```python
from build123d import *

# Parameters (mm, degrees)
F0_W     = 22
F0_H     = 55
F1_DEPTH = 3
F2_R     = 2
F4_DEPTH = 2
F5_R     = 4
F6_R     = 19
F6_R_2   = 16.5
F7_DEPTH = 15
F9_DEPTH = 25


with BuildPart() as f1:
    # F0 (on Top) → F1 (new body)
    with BuildSketch(Plane.XY):
        Rectangle(F0_W, F0_H)
    extrude(amount=F1_DEPTH)

    # F2
    f2_edges = [f1.edges().sort_by_distance(p)[0] for p in [
        (-11, 27.5, 1.5),
        (11, 27.5, 1.5),
        (11, -27.5, 1.5),
        (-11, -27.5, 1.5),
    ]]
    fillet(f2_edges, radius=F2_R)

    # F3 (on face) → F4 (join)
    with BuildSketch(Plane.XZ.offset(27.5)):
        with BuildLine():
            Line((-9, 3), (-4.24e-08, 3))
            Line((-4.24e-08, 3), (9, 3))
            Line((9, 3), (9, 2.7667994693))
            ThreePointArc((9, 2.7667994693), (16.3095064303, 9.7532056552), (19, 19.5))
            ThreePointArc((19, 19.5), (-9.7467943448, 35.8095064303), (-9, 2.7667994693))
            Line((-9, 2.7667994693), (-9, 3))
        make_face()
        with BuildLine():
            ThreePointArc((-4.24e-08, 3), (-11.6672618746, 31.1672619046), (16.5, 19.5))
            ThreePointArc((16.5, 19.5), (11.6672618746, 7.8327380954), (-4.24e-08, 3))
        make_face(mode=Mode.SUBTRACT)
        with BuildLine():
            ThreePointArc((-4.24e-08, 3), (11.6672618746, 7.8327380954), (16.5, 19.5))
            ThreePointArc((16.5, 19.5), (-11.6672618746, 31.1672619046), (-4.24e-08, 3))
        make_face()
    extrude(amount=-F4_DEPTH)

    # F5
    f5_edges = [f1.edges().sort_by_distance(p)[0] for p in [
        (0, -25.5, 3),
    ]]
    fillet(f5_edges, radius=F5_R)

    # F6 (on face) → F7 (join)
    with BuildSketch(Plane(origin=(0, 27.5, 0), x_dir=(-1, 0, 0), z_dir=(0, 1, 0))):
        with Locations((0, 19.5)):
            Circle(F6_R)
        with Locations((0, 19.5)):
            Circle(F6_R_2, mode=Mode.SUBTRACT)
    extrude(amount=-F7_DEPTH)

    # F8 (on face) → F9 (cut)
    with BuildSketch(Plane(origin=(0, 27.5, 0), x_dir=(-1, 0, 0), z_dir=(0, 1, 0))):
        Polygon((-10.5, 26.4886836855), (0, 26.4886836855), (10.5, 26.4886836855), (23.2279220614, 39.2166057468), (-23.2279220614, 39.2166057468), align=None)
    extrude(amount=-F9_DEPTH, mode=Mode.SUBTRACT)


solid = f1.part
```
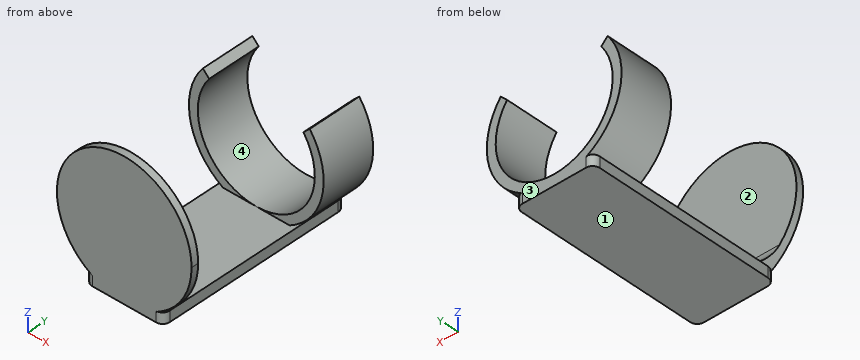
Verification items for the finished model (mm, model axes). Face numbers are marked on the shaded views. A direction names the side the tool comes from. Coordinates: 2 decimals unless noted, no trailing zeros. Loops run counter-clockwise (first coordinate to the right, second up) from the corner with the lowest first, then second, coordinate; pieces in that order, holes last. Notation, with made-up numbers: (5.5, 47.5) -> (38.5, 47.5) arc R22 ccw to (38.5, 77.5) -> close; hole circle Ø1 at (85, 5). An arc over 180 degrees is marked (long way). Answer in a Markdown table with one row per item.
1) Draft check along X on the marked faces 3 and 4. Enter one of: released by +X, released by -X, zero draft, split by the parting line, or undercut.
The answers:
| item | result |
|---|---|
| face 3 | zero draft |
| face 4 | undercut |
2) Section check D-D (z = 34). Record the cut outline in (x, y), and give its area (3 significant figures).
The answers:
| item | result |
|---|---|
| outline | (-12.28, -27.5) -> (12.28, -27.5) -> (12.28, -25.5) -> (-12.28, -25.5) -> close |
| area | 49.1 mm2 |
3) Section check C-C (y = 14). Record the cut outline in (x, z).
The answers:
| item | result |
|---|---|
| outline | (-15.08, 31.06) arc R19 ccw to (-9.42, 3) -> (-11, 3) -> (-11, 0) -> (11, 0) -> (11, 3) -> (9.42, 3) arc R19 ccw to (15.08, 31.06) -> (13.29, 29.28) arc R16.5 cw (long way) to (-13.29, 29.28) -> close |
4) Scan lines: line 1 along X through (y, z) = (24, 19.5); line 2 along Z through (x, y) = (0, 16); line 3 along Y through (x, z) = (-10, 9). Record each from-to range of solid material in increasing order. Write a range as from..to.
The answers:
| item | result |
|---|---|
| line 1 | x = -19..-16.5, 16.5..19 |
| line 2 | z = 0..3 |
| line 3 | y = -27.5..-25.5 |
5) Section check A-A (z = 22.5). Record the cut outline in (x, y).
The answers:
| item | result |
|---|---|
| outline | (-18.76, -27.5) -> (18.76, -27.5) -> (18.76, -25.5) -> (-18.76, -25.5) -> close; (-18.76, 12.5) -> (-16.22, 12.5) -> (-16.22, 27.5) -> (-18.76, 27.5) -> close; (16.22, 12.5) -> (18.76, 12.5) -> (18.76, 27.5) -> (16.22, 27.5) -> close |
6) Depth check by flat-ended pin: P1, Ø0.9, axis at y = 2.5, z = 1, coming from the -X side; P2, Ø5, axis at x = -0.5, z = 17, coming from the +Y side; P3, Ø10, axis at x = -2, y = -1, coming from the +Z side. Enter the tip coordinate at first touch or a pass-through.
The answers:
| item | result |
|---|---|
| P1 | stops at x = -11 |
| P2 | stops at y = -25.5 |
| P3 | stops at z = 3 |
7) Section check B-B (x = -4). Record the cut outline in (y, z).
The answers:
| item | result |
|---|---|
| outline | (-27.5, 0) -> (27.5, 0) -> (27.5, 3.49) -> (12.5, 3.49) -> (12.5, 3) -> (-21.5, 3) arc R4 cw to (-25.5, 7) -> (-25.5, 38.07) -> (-27.5, 38.07) -> close |
8) Access from +Z, -Z, +X, -X, +Y, -Y to the whole of each face (thin tool, end or side, straight path). Record for the marked faces 1 and 2.
The answers:
| item | result |
|---|---|
| face 1 | -Z, +X, -X, +Y, -Y |
| face 2 | +Z, +X, -X |
